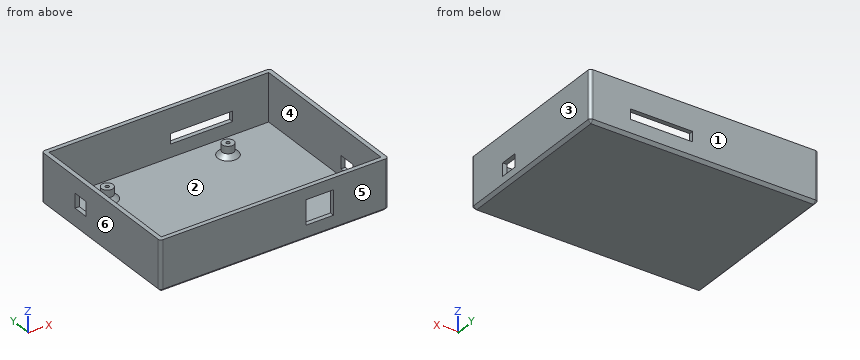
from build123d import *

# Parameters (mm, degrees)
SKETCH010_W     = 158
SKETCH010_H     = 118
PAD003_DEPTH    = 35
SKETCH011_W     = 152
SKETCH011_H     = 112
POCKET006_DEPTH = 33
SKETCH012_R     = 4
SKETCH012_R_2   = 1.25
PAD004_DEPTH    = 8
CHAMFER_SIZE    = 3
SKETCH013_W     = 10.869108
SKETCH013_H     = 10
POCKET007_DEPTH = 3
SKETCH014_W     = 19
SKETCH014_H     = 17
POCKET008_DEPTH = 3.001
SKETCH015_W     = 43
SKETCH015_H     = 7
POCKET009_DEPTH = 3.001
FILLET_R        = 2
CHAMFER001_SIZE = 2
SKETCH019_W     = 12
SKETCH019_H     = 9
POCKET012_DEPTH = 3.001


with BuildPart() as part:
    # Sketch010 (on XY_Plane176 of Origin352) → Pad003 (new body)
    with BuildSketch(Plane.XY):
        with Locations((15.5, -8.25)):
            Rectangle(SKETCH010_W, SKETCH010_H)
    extrude(amount=PAD003_DEPTH)

    # Sketch011 (on Face6 of Pad003) → Pocket006 (cut)
    with BuildSketch(Plane.XY.offset(35)):
        with Locations((15.5, -8.25)):
            Rectangle(SKETCH011_W, SKETCH011_H)
    extrude(amount=-POCKET006_DEPTH, mode=Mode.SUBTRACT)

    # Sketch012 (on Face11 of Pocket006) → Pad004 (join)
    with BuildSketch(Plane.XY.offset(2)):
        with Locations((-31.25, 31.75)):
            Circle(SKETCH012_R)
        with Locations((-31.25, 31.75)):
            Circle(SKETCH012_R_2, mode=Mode.SUBTRACT)
        with Locations((52.25, 31.75)):
            Circle(SKETCH012_R)
        with Locations((52.25, 31.75)):
            Circle(SKETCH012_R_2, mode=Mode.SUBTRACT)
        with Locations((73.75, -52.25)):
            Circle(SKETCH012_R)
        with Locations((73.75, -52.25)):
            Circle(SKETCH012_R_2, mode=Mode.SUBTRACT)
        with Locations((-31.25, -42.25)):
            Circle(SKETCH012_R)
        with Locations((-31.25, -42.25)):
            Circle(SKETCH012_R_2, mode=Mode.SUBTRACT)
    extrude(amount=PAD004_DEPTH)

    # Chamfer
    chamfer_edges = [part.edges().sort_by_distance(p)[0] for p in [
        (48.25, 31.75, 2),
        (-35.25, 31.75, 2),
        (-35.25, -42.25, 2),
        (69.75, -52.25, 2),
    ]]
    chamfer(chamfer_edges, length=CHAMFER_SIZE)

    # Sketch013 (on Face3 of Chamfer) → Pocket007 (cut)
    with BuildSketch(Plane.YZ.offset(-60.5)):
        with Locations((12.019298, 19)):
            Rectangle(SKETCH013_W, SKETCH013_H)
    extrude(amount=-POCKET007_DEPTH, mode=Mode.SUBTRACT)

    # Sketch014 (on Face5 of Pocket007) → Pocket008 (cut, through all)
    with BuildSketch(Plane(origin=(0, -64.25, 0), x_dir=(-1, 0, 0), z_dir=(0, 1, 0))):
        with Locations((-47, 18.5)):
            Rectangle(SKETCH014_W, SKETCH014_H)
    extrude(amount=-POCKET008_DEPTH, mode=Mode.SUBTRACT)

    # Sketch015 (on Face4 of Pocket008) → Pocket009 (cut, through all)
    with BuildSketch(Plane.XZ.offset(-47.75)):
        with Locations((45, 14.5)):
            Rectangle(SKETCH015_W, SKETCH015_H)
    extrude(amount=-POCKET009_DEPTH, mode=Mode.SUBTRACT)

    # Fillet
    fillet_edges = [part.edges().sort_by_distance(p)[0] for p in [
        (94.5, -67.25, 17.5),
        (-63.5, -67.25, 17.5),
        (-63.5, 50.75, 17.5),
        (94.5, 50.75, 17.5),
    ]]
    fillet(fillet_edges, radius=FILLET_R)

    # Chamfer001
    chamfer001_edges = [part.edges().sort_by_distance(p)[0] for p in [
        (94.5, -8.25, 0),
        (15.5, 50.75, 0),
        (-63.5, -8.25, 0),
        (15.5, -67.25, 0),
    ]]
    chamfer(chamfer001_edges, length=CHAMFER001_SIZE)

    # Sketch019 (on Face20 of Chamfer001) → Pocket012 (cut, through all)
    with BuildSketch(Plane(origin=(91.5, 0, 0), x_dir=(0, -1, 0), z_dir=(-1, 0, 0))):
        with Locations((30.25, 11.5)):
            Rectangle(SKETCH019_W, SKETCH019_H)
    extrude(amount=-POCKET012_DEPTH, mode=Mode.SUBTRACT)


solid = part.part
Verification items for the finished model (mm, model axes). Face numbers are marked on the shaded views. A direction names the side the tool comes from. Give positions to 0.01 mm unless a question says otherwise; leave off trailing zeros. Order: outer loops, then holes, each group sorted by start corner. A loop starts at its lowest first (then second) coordinate and runs counter-clockwise, first axis right, second up. Notation, with made-up numbers: M -29.5,14.25 L 24.5,14.25 A26 cw 24.5,50.25 Z; hole C -11,6.25 d2. An arc over 180 degrees is marked long. Use one line per item in the form item = value. Start each with the question number.
Q1. Access from +Z, -Z, +X, -X, +Y, -Y to the whole of each face (thin tool, end or side, straight path). Record for the marked faces 1 and 2.
Q2. Section check D-D (x = -8). Enter the section's corners in (y, z), then the cut area to 3 significant figures.
Q3. Section check A-A (y = -29). Enter the section's corners in (x, z).
Q4. Mould release check, pull along X, two halves, no side actions. Record for the marked faces 3, 4, 5 and 6: +X half, -X half, draft (parallel to the pull), parting line (faces both ways), or undercut.
Q5. Scan lines: line 1 along Y through (x, z) = (-31.25, 8.25); line 2 along X through (y, z) = (36, 7.5); line 3 along Y through (x, z) = (37.5, 4). Record each from-to range of solid material in increasing order. Write a range as [from, to].
Q6. Go/stop test with flat-tipped pins: pin 1 Ø1.2 at (x, y) = (-31.5, -42) entering from +Z; pin 2 Ø1.5 at (y, z) = (49, 15.5) entering from -X; pin 3 Ø6.5 at (x, y) = (53, 33.5) entering from +Z. Record where each tip stops, or that it passes through.
Q7. Section check B-B (x = 34). Enter the section's corners in (y, z), then the cut area to 3 significant figures.
Q8. Section check C-C (y = -4.5). Enter the section's corners in (x, z).
Evaluation:
q1.face_1 = +Z, -Z, +X, -X, +Y
q1.face_2 = +Z
q2.outline = M -67.25,2 L -65.25,0 L 48.75,0 L 50.75,2 L 50.75,35 L 47.75,35 L 47.75,2 L -64.25,2 L -64.25,35 L -67.25,35 Z
q2.area = 430 mm2
q3.outline = M -63.5,2 L -61.5,0 L 92.5,0 L 94.5,2 L 94.5,7 L 91.5,7 L 91.5,2 L -60.5,2 L -60.5,35 L -63.5,35 Z; M 91.5,16 L 94.5,16 L 94.5,35 L 91.5,35 Z
q4.face_3 = +X half
q4.face_4 = undercut
q4.face_5 = draft
q4.face_6 = -X half
q5.line_1 = [-67.25, -64.25], [-46.25, -43.5], [-41, -38.25], [27.75, 30.5], [33, 35.75], [47.75, 50.75]
q5.line_2 = [-63.5, -60.5], [91.5, 94.5]
q5.line_3 = [-67.25, -64.25], [47.75, 50.75]
q6.pin_1 = 2
q6.pin_2 = -63.5
q6.pin_3 = 10
q7.outline = M -67.25,2 L -65.25,0 L 48.75,0 L 50.75,2 L 50.75,11 L 47.75,11 L 47.75,2 L -64.25,2 L -64.25,35 L -67.25,35 Z; M 47.75,18 L 50.75,18 L 50.75,35 L 47.75,35 Z
q7.area = 409 mm2
q8.outline = M -63.5,2 L -61.5,0 L 92.5,0 L 94.5,2 L 94.5,35 L 91.5,35 L 91.5,2 L -60.5,2 L -60.5,35 L -63.5,35 Z
